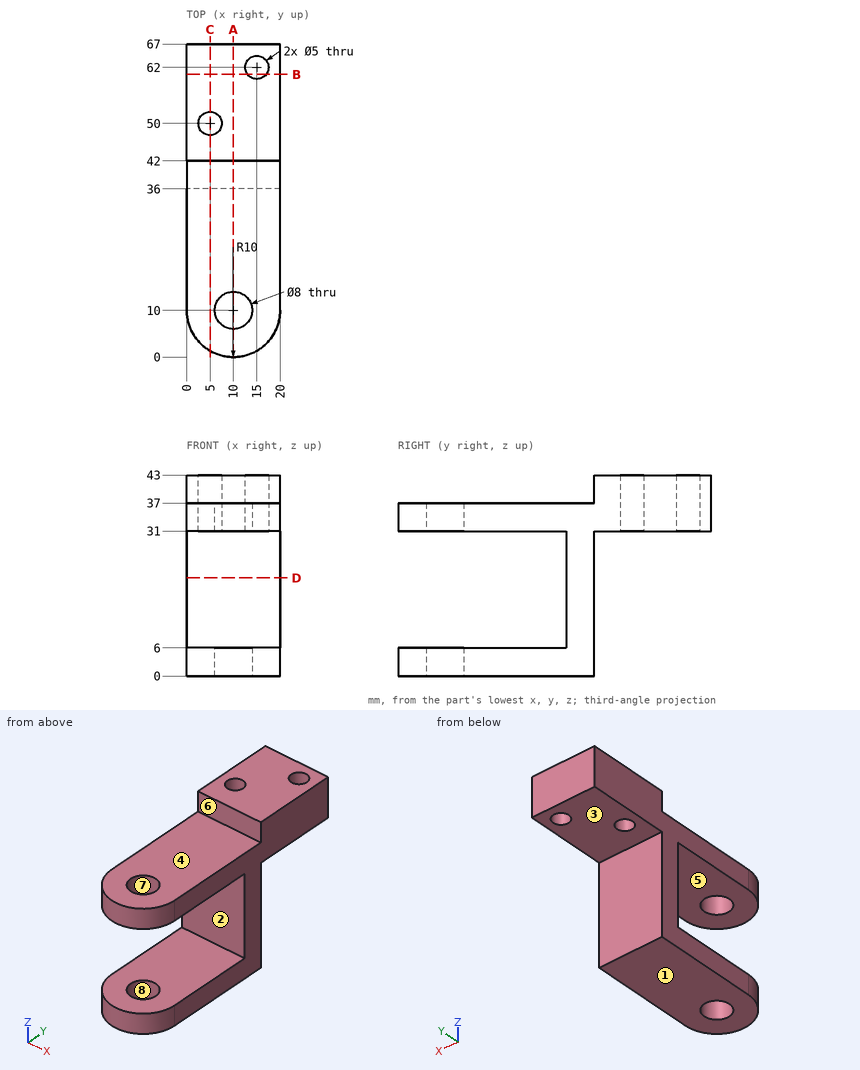
The drawing under review shows one solid part. Ordinate dimensions are in mm from its lowest x, y, z. A direction names the side the tool comes from. Coordinates: 2 decimals unless noted, no trailing zeros. Write each loop counter-clockwise with the first axis right and the second up, starting at its lowest first coordinate (ties: lowest second). Pieces come first, ordered by that corner, then holes. Notation, with made-up numbers: (-40, -32.5) -> (-34, -32.5) arc R35 cw to (-34, 2.5) -> close; hole circle Ø8 at (44, -38.75). An arc over 180 degrees is marked (long way). One line per item, written item: value. Start each with the question number.
Q1. For the marked faces 1, 2, 3 and 4, list the 3-axis set-ups (+Z, -Z, +X, -X, +Y, -Y) from which the entire face can be reached by the end or side of a thin tool; tool diameter is ignored.
Q2. Add section C-C, the plane x = 5. Give the boundary of the cut face in (y, z).
Q3. The part is to be moulded in two halves that separate along Y. For the marked faces 5, 6, 7 and 8, say which applies: +Y half, -Y half, draft (parallel to the pull), parting line (faces both ways), or undercut.
Q4. Add section D-D, the plane z = 21. Give the boundary of the cut face in (x, y).
Q5. Add section A-A, the plane x = 10. Give the boundary of the cut face in (y, z), then the cut area to 3 significant figures.
Q6. Add section B-B, the plane y = 60.5. Give the boundary of the cut face in (x, z).
Q7. To check wall thickness, follow probe 1 along Z at (x, y) = (4.5, 26); probe 2 along Y at (x, z) = (10, 3.45); probe 3 along Y at (x, z) = (10, 34.8). State the ranges of each line that lie inside material, in increasing order.
Q8. Clearance check with flat-ended pins moving along their axes: P1, Ø6, axis at x = 14.5, y = 53, coming from the -Z side; P2, Ø1, axis at x = 4.5, z = 12, coming from the +Y side; P3, Ø1, axis at x = 2, y = 24, coming from the +Z side. State where each tip first meets the part, or that it passes through.
Response:
1. face 1: -Z, +X, -X, +Y, -Y
1. face 2: +X, -X, -Y
1. face 3: -Z, +X, -X, +Y
1. face 4: +Z, +X, -X, -Y
2. outline: (1.34, 0) -> (42, 0) -> (42, 31) -> (47.5, 31) -> (47.5, 43) -> (42, 43) -> (42, 37) -> (1.34, 37) -> (1.34, 31) -> (36, 31) -> (36, 6) -> (1.34, 6) -> close; (52.5, 31) -> (67, 31) -> (67, 43) -> (52.5, 43) -> close
3. face 5: draft
3. face 6: -Y half
3. face 7: undercut
3. face 8: undercut
4. outline: (0, 36) -> (20, 36) -> (20, 42) -> (0, 42) -> close
5. outline: (0, 0) -> (6, 0) -> (6, 6) -> (0, 6) -> close; (0, 31) -> (6, 31) -> (6, 37) -> (0, 37) -> close; (14, 0) -> (42, 0) -> (42, 31) -> (67, 31) -> (67, 43) -> (42, 43) -> (42, 37) -> (14, 37) -> (14, 31) -> (36, 31) -> (36, 6) -> (14, 6) -> close
5. area: 858 mm²
6. outline: (0, 31) -> (13, 31) -> (13, 43) -> (0, 43) -> close; (17, 31) -> (20, 31) -> (20, 43) -> (17, 43) -> close
7. probe 1: 0 to 6, 31 to 37
7. probe 2: 0 to 6, 14 to 42
7. probe 3: 0 to 6, 14 to 67
8. P1: z = 31
8. P2: y = 42
8. P3: z = 37
